```python
from build123d import *

# Parameters (mm, degrees)
SKETCH1_W                        = 38.1
SKETCH1_H                        = 38.1
SKETCH1_W_2                      = 31.75
SKETCH1_H_2                      = 31.75
BOSS_EXTRUDE1_DEPTH              = 203.2
SKETCH3_W                        = 2.4892
SKETCH3_H                        = 3.175
SKETCH3_AT_POINT_2_W             = 2.4892
SKETCH3_AT_POINT_2_H             = 3.175
SKETCH3_AT_POINT_3_W             = 2.4892
SKETCH3_AT_POINT_3_H             = 3.175
F_3_8_0_375_DIAMETER_HOLE1_D     = 9.525
F_3_8_0_375_DIAMETER_HOLE1_DEPTH = 3.175
LPATTERN1_START                  = 15.875
LPATTERN1_OUTLINE_R              = 4.7625
LPATTERN1_DEPTH                  = 3.175
LPATTERN1_START_2                = -19.05
LPATTERN1_2_OUTLINE_R            = 2.4892
LPATTERN1_2_DEPTH                = 3.175
LPATTERN1_3_OUTLINE_R            = 2.4892
LPATTERN1_3_DEPTH                = 38.1


# Read off the part's stored shape, not the designer's step: LPattern1
with BuildPart() as part:
    # Sketch1 → Boss-Extrude1 (new, symmetric)
    with BuildSketch(Plane(origin=(0, 0, 0), x_dir=(0, 0, -1), z_dir=(1, 0, 0))):
        Rectangle(SKETCH1_W, SKETCH1_H)
        Rectangle(SKETCH1_W_2, SKETCH1_H_2, mode=Mode.SUBTRACT)
    extrude(amount=BOSS_EXTRUDE1_DEPTH, both=True)

    # Sketch3 → #9 (0.196) Diameter Hole1 (revolve, cut)
    with BuildSketch(Plane(origin=(190.5, 19.05, 0), x_dir=(0, 0, 1), z_dir=(1, 0, 0))):
        with Locations((1.2446, 1.5875)):
            Rectangle(SKETCH3_W, SKETCH3_H)
    revolve(axis=Axis((190.5, 25.4, 0), (0, -1, 0)), mode=Mode.SUBTRACT)

    # Sketch3 at point 2 (carried to point 2, square into its face) → #9 (0.196) Diameter Hole1 at 2 (revolve, cut)
    with BuildSketch(Plane(origin=(190.5, -19.05, 0), x_dir=(0, 0, 1), z_dir=(-1, 0, 0))):
        with Locations((1.2446, 1.5875)):
            Rectangle(SKETCH3_AT_POINT_2_W, SKETCH3_AT_POINT_2_H)
    revolve(axis=Axis((190.5, -25.4, 0), (0, 1, 0)), mode=Mode.SUBTRACT)

    # Sketch3 at point 3 (carried to point 3, square into its face) → #9 (0.196) Diameter Hole1 at 3 (revolve, cut)
    with BuildSketch(Plane(origin=(190.5, 0, -19.05), x_dir=(0, 1, 0), z_dir=(1, 0, 0))):
        with Locations((1.2446, 1.5875)):
            Rectangle(SKETCH3_AT_POINT_3_W, SKETCH3_AT_POINT_3_H)
    revolve(axis=Axis((190.5, 0, -25.4), (0, 0, 1)), mode=Mode.SUBTRACT)

    # 3/8 (0.375) Diameter Hole1
    with Locations(Plane(origin=(190.5, 0, 19.05), x_dir=(1, 0, 0), z_dir=(0, 0, 1))):
        with Locations((0, 0)):
            Hole(F_3_8_0_375_DIAMETER_HOLE1_D / 2, depth=F_3_8_0_375_DIAMETER_HOLE1_DEPTH)

    # LPattern1 outline → LPattern1 (cut)
    with BuildSketch(Plane.XY.offset(LPATTERN1_START)):
        with Locations((165.1, 0)):
            Circle(LPATTERN1_OUTLINE_R)
        with Locations((139.7, 0)):
            Circle(LPATTERN1_OUTLINE_R)
        with Locations((114.3, 0)):
            Circle(LPATTERN1_OUTLINE_R)
        with Locations((88.9, 0)):
            Circle(LPATTERN1_OUTLINE_R)
        with Locations((63.5, 0)):
            Circle(LPATTERN1_OUTLINE_R)
        with Locations((38.1, 0)):
            Circle(LPATTERN1_OUTLINE_R)
        with Locations((12.7, 0)):
            Circle(LPATTERN1_OUTLINE_R)
        with Locations((-12.7, 0)):
            Circle(LPATTERN1_OUTLINE_R)
        with Locations((-38.1, 0)):
            Circle(LPATTERN1_OUTLINE_R)
        with Locations((-63.5, 0)):
            Circle(LPATTERN1_OUTLINE_R)
        with Locations((-88.9, 0)):
            Circle(LPATTERN1_OUTLINE_R)
        with Locations((-114.3, 0)):
            Circle(LPATTERN1_OUTLINE_R)
        with Locations((-139.7, 0)):
            Circle(LPATTERN1_OUTLINE_R)
        with Locations((-165.1, 0)):
            Circle(LPATTERN1_OUTLINE_R)
        with Locations((-190.5, 0)):
            Circle(LPATTERN1_OUTLINE_R)
    extrude(amount=LPATTERN1_DEPTH, mode=Mode.SUBTRACT)

    # LPattern1 2 outline → LPattern1 2 (cut)
    with BuildSketch(Plane.XY.offset(LPATTERN1_START_2)):
        with Locations((165.1, 0)):
            Circle(LPATTERN1_2_OUTLINE_R)
        with Locations((139.7, 0)):
            Circle(LPATTERN1_2_OUTLINE_R)
        with Locations((114.3, 0)):
            Circle(LPATTERN1_2_OUTLINE_R)
        with Locations((88.9, 0)):
            Circle(LPATTERN1_2_OUTLINE_R)
        with Locations((63.5, 0)):
            Circle(LPATTERN1_2_OUTLINE_R)
        with Locations((38.1, 0)):
            Circle(LPATTERN1_2_OUTLINE_R)
        with Locations((12.7, 0)):
            Circle(LPATTERN1_2_OUTLINE_R)
        with Locations((-12.7, 0)):
            Circle(LPATTERN1_2_OUTLINE_R)
        with Locations((-38.1, 0)):
            Circle(LPATTERN1_2_OUTLINE_R)
        with Locations((-63.5, 0)):
            Circle(LPATTERN1_2_OUTLINE_R)
        with Locations((-88.9, 0)):
            Circle(LPATTERN1_2_OUTLINE_R)
        with Locations((-114.3, 0)):
            Circle(LPATTERN1_2_OUTLINE_R)
        with Locations((-139.7, 0)):
            Circle(LPATTERN1_2_OUTLINE_R)
        with Locations((-165.1, 0)):
            Circle(LPATTERN1_2_OUTLINE_R)
        with Locations((-190.5, 0)):
            Circle(LPATTERN1_2_OUTLINE_R)
    extrude(amount=LPATTERN1_2_DEPTH, mode=Mode.SUBTRACT)

    # LPattern1 3 outline → LPattern1 3 (cut)
    with BuildSketch(Plane(origin=(0, 0, 0), x_dir=(1, 0, 0), z_dir=(0, 1, 0)).offset(LPATTERN1_START_2)):
        with Locations((165.1, 0)):
            Circle(LPATTERN1_3_OUTLINE_R)
        with Locations((139.7, 0)):
            Circle(LPATTERN1_3_OUTLINE_R)
        with Locations((114.3, 0)):
            Circle(LPATTERN1_3_OUTLINE_R)
        with Locations((88.9, 0)):
            Circle(LPATTERN1_3_OUTLINE_R)
        with Locations((63.5, 0)):
            Circle(LPATTERN1_3_OUTLINE_R)
        with Locations((38.1, 0)):
            Circle(LPATTERN1_3_OUTLINE_R)
        with Locations((12.7, 0)):
            Circle(LPATTERN1_3_OUTLINE_R)
        with Locations((-12.7, 0)):
            Circle(LPATTERN1_3_OUTLINE_R)
        with Locations((-38.1, 0)):
            Circle(LPATTERN1_3_OUTLINE_R)
        with Locations((-63.5, 0)):
            Circle(LPATTERN1_3_OUTLINE_R)
        with Locations((-88.9, 0)):
            Circle(LPATTERN1_3_OUTLINE_R)
        with Locations((-114.3, 0)):
            Circle(LPATTERN1_3_OUTLINE_R)
        with Locations((-139.7, 0)):
            Circle(LPATTERN1_3_OUTLINE_R)
        with Locations((-165.1, 0)):
            Circle(LPATTERN1_3_OUTLINE_R)
        with Locations((-190.5, 0)):
            Circle(LPATTERN1_3_OUTLINE_R)
    extrude(amount=LPATTERN1_3_DEPTH, mode=Mode.SUBTRACT)


solid = part.part
```
Could you check a few things on this model? Use its own coordinates, in mm. A direction names the side the tool comes from. Give positions to 0.01 mm unless a question says otherwise; leave off trailing zeros. Loops run counter-clockwise (first coordinate to the right, second up) from the corner with the lowest first, then second, coordinate; pieces in that order, holes last. Notation, with made-up numbers: (85.25, 43) -> (91.25, 43) arc R16 ccw to (91.25, 48) -> close; hole circle Ø3 at (78.5, 27). An arc over 180 degrees is marked (long way). Put each result on its own line as item: value.
(1) Please list where these lines run through material, in increasing order: probe 1 along Z at (x, y) = (104.5, -11) (3 decimals); probe 2 along Y at (x, z) = (-114, -16). Write a range as [from, to].
Computed:
probe 1: [-19.05, -15.875], [15.875, 19.05]
probe 2: [-19.05, -2.47], [2.47, 19.05]
(2) Imagine slicing it at B-B on x = 130.5. Write out the boundary of the cut face in (y, z) (3 decimals), plus the area to 3 significant figures.
Computed:
outline: (-19.05, -19.05) -> (19.05, -19.05) -> (19.05, 19.05) -> (-19.05, 19.05) -> close; hole (-15.875, -15.875) -> (15.875, -15.875) -> (15.875, 15.875) -> (-15.875, 15.875) -> close
area: 444 mm^2
(3) Imagine slicing it at A-A on z = -7. Write out the boundary of the cut face in (x, y) (3 decimals).
Computed:
outline: (-203.2, -19.05) -> (203.2, -19.05) -> (203.2, -15.875) -> (-203.2, -15.875) -> close; (-203.2, 15.875) -> (203.2, 15.875) -> (203.2, 19.05) -> (-203.2, 19.05) -> close
(4) For faces 4 (the face through (3, 0, 15.875)), 5 (the face through (3, 0, 19.05)), 6 (the face through (195.258, 0.209, 17.44)), which set-ups out of +Z, -Z, +X, -X, +Y, -Y let a thin tool reach every point of the face, with its end or its side?
Computed:
face 4: +X, -X
face 5: +Z, +X, -X, +Y, -Y
face 6: +Z
(5) Thinking about a two-plate mould opening in Y: for faces 1 (the face through (3, 0, -19.05)), 2 (the face through (3, -19.05, 0)), 3 (the face through (118.843, 1.431, 17.44)), which applies, pulls with the +Y half, pulls with the -Y half, needs draft (parallel to the pull), parting line crosses it, or undercut?
Computed:
face 1: needs draft
face 2: pulls with the -Y half
face 3: undercut
(6) I'm going to push flat-ended pins straight in: pin 1 Ø4 at (y, z) = (-12.5, -5) entering from -X; pin 2 Ø5.5 at (x, y) = (190.5, 0) entering from +Z (3 decimals). Where does each tip first touch, or does it pass through?
Computed:
pin 1: through
pin 2: z = -15.875
